```python
from build123d import *

# Parameters (mm, degrees)
SKETCH1_R           = 15
BOSS_EXTRUDE1_DEPTH = 25
BOSS_EXTRUDE2_START = 5
BOSS_EXTRUDE2_DEPTH = 5


with BuildPart() as part:
    # Sketch1 → Boss-Extrude1 (new body)
    with BuildSketch(Plane(origin=(0, 0, 0), x_dir=(1, 0, 0), z_dir=(0, 1, 0))):
        with BuildLine():
            Line((-32.5, -45), (-32.5, -55))
            Line((-32.5, -55), (32.5, -55))
            Line((32.5, -55), (32.5, -45))
            Line((32.5, -45), (5, -45))
            Line((5, -45), (5, -21.937410968))
            ThreePointArc((5, -21.937410968), (0, 22.5), (-5, -21.937410968))
            Line((-5, -21.937410968), (-5, -45))
            Line((-5, -45), (-32.5, -45))
        make_face()
        with Locations(Location((0, 0, 0), (0, 0, 270))):
            Circle(SKETCH1_R, mode=Mode.SUBTRACT)
    extrude(amount=BOSS_EXTRUDE1_DEPTH)

    # Sketch1<3> → Boss-Extrude2 (add)
    with BuildSketch(Plane(origin=(0, 0, 0), x_dir=(1, 0, 0), z_dir=(0, 1, 0)).offset(BOSS_EXTRUDE2_START)):
        with BuildLine():
            ThreePointArc((24.904867452, 2.178893569), (0, 25), (-24.904867452, 2.178893569))
            Line((-24.904867452, 2.178893569), (-29.032485797, -45))
            Line((-29.032485797, -45), (-5, -45))
            Line((-5, -45), (-5, -24.494897428))
            Line((-5, -24.494897428), (-5, -21.937410968))
            ThreePointArc((-5, -21.937410968), (-14.0312152, 17.589059099), (22.5, 0))
            ThreePointArc((22.5, 0), (17.589059099, -14.0312152), (5, -21.937410968))
            Line((5, -21.937410968), (5, -24.494897428))
            Line((5, -24.494897428), (5, -45))
            Line((5, -45), (29.032485797, -45))
            Line((29.032485797, -45), (24.904867452, 2.178893569))
        make_face()
    extrude(amount=BOSS_EXTRUDE2_DEPTH)


solid = part.part
```
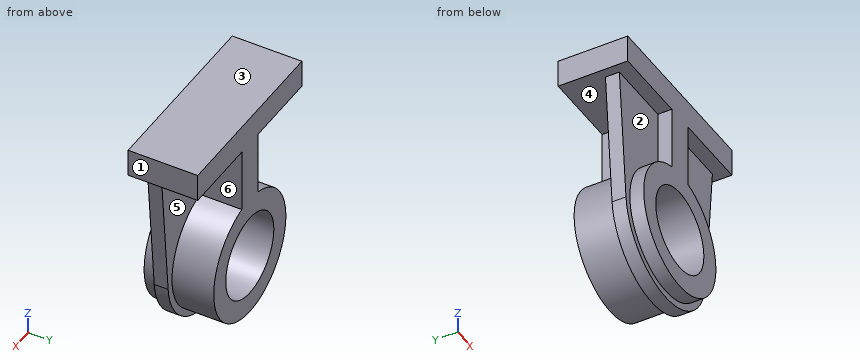
Read the model definition and answer for the solid it produces. Units are mm, in the model's axes. Face numbers are marked on the shaded views. A direction names the side the tool comes from. Coordinates: 2 decimals unless noted, no trailing zeros. Order: outer loops, then holes, each group sorted by start corner. A loop starts at its lowest first (then second) coordinate and runs counter-clockwise, first axis right, second up. Notation, with made-up numbers: (-31, -22.75) - (-15, -22.75) arc R27 cw to (-15, 14.25) - close; hole circle Ø5 at (5, -21). An arc over 180 degrees is marked (long way). Answer as a JSON object with one key per item and string values. Group by question number.
Item 1: A tool of negligible diameter and unlimited length cuts with its end or side. For the marked faces 4, 5 and 6, from which of +Z, -Z, +X, -X, +Y, -Y can it reach the whole face along a straight path? Write none if from no direction.
Item 2: Section A-A (x = 0) is taken. Give the vertices of the cut face in (y, z).
Item 3: Section C-C (z = 12) is taken. Give the vertices of the cut face in (x, y).
Item 4: Section B-B (y = 2.25) is taken. Give the vertices of the cut face in (x, z), plus the area to 3 significant figures.
Item 5: Consider probe 1 along X at (y, z) = (10.5, 0); probe 2 along Z at (x, y) = (-6.5, 4.5); probe 3 along X at (y, z) = (15.5, 28.5). Determine where each line is inside the solid, lowest interval first. Write a range as from..to.
Item 6: Section D-D (y = 8.5) is taken. Give the vertices of the cut face in (x, z).
Item 7: Flat-ended cylindrical pins translate along their axes: P1, Ø1, axis at x = -4.5, y = 11, coming from the -Z side; P2, Ø12.5, axis at x = -16.5, y = 18, coming from the -Z side; P3, Ø2, axis at x = 14, y = 16.5, coming from the -Z side. Find the tip coordinate at first contact, or state that the pin passes through.
Item 8: The mould has two halves that part along Z. Classify the marked faces 1, 2 and 3: +Z half, -Z half, draft (parallel to the pull), parting line (faces both ways), or undercut.
Results are:
{
 "1": {"face 4": "-X", "face 5": "+Y", "face 6": "+X, +Y"},
 "2": {"outline": "(0, -22.5) - (5, -22.5) - (5, -25) - (10, -25) - (10, -22.5) - (25, -22.5) - (25, -15) - (0, -15) - close; (0, 15) - (25, 15) - (25, 55) - (0, 55) - close"},
 "3": {"outline": "(-26.15, 5) - (-19.03, 5) - (-19.03, 0) - (-9, 0) - (-9, 25) - (-19.03, 25) - (-19.03, 10) - (-26.15, 10) - close; (9, 0) - (19.03, 0) - (19.03, 5) - (26.15, 5) - (26.15, 10) - (19.03, 10) - (19.03, 25) - (9, 25) - close"},
 "4": {"outline": "(-32.5, 45) - (-5, 45) - (-5, 21.94) arc R22.5 ccw (long way) to (5, 21.94) - (5, 45) - (32.5, 45) - (32.5, 55) - (-32.5, 55) - close; hole circle Ø30 at (0, 0)", "area": "1,760 mm^2"},
 "5": {"probe 1": "x = -22.5..-15, 15..22.5", "probe 2": "z = -21.54..-13.52, 13.52..21.54, 45..55", "probe 3": "x = -5..5"},
 "6": {"outline": "(-32.5, 45) - (-29.03, 45) - (-24.9, -2.18) arc R25 ccw to (24.9, -2.18) - (29.03, 45) - (32.5, 45) - (32.5, 55) - (-32.5, 55) - close; hole circle Ø30 at (0, 0)"},
 "7": {"P1": "stops at z = -22.14", "P2": "stops at z = -20.03", "P3": "stops at z = -18.36"},
 "8": {"face 1": "draft", "face 2": "undercut", "face 3": "+Z half"}
}
